Can you work these out from the drawing? Everything is in mm from the part's minimum corner. Round coordinates to 2 decimals unless told otherwise and drop trailing zeros. Loops run counter-clockwise (first coordinate to the right, second up) from the corner with the lowest first, then second, coordinate; pieces in that order, holes last. Notation, with made-up numbers: (-26, -10) -> (-10, -10) arc R21 cw to (-10, 24) -> close; hole circle Ø11 at (38, -14.5). An arc over 180 degrees is marked (long way). Answer as a JSON object with one key per item and string values.
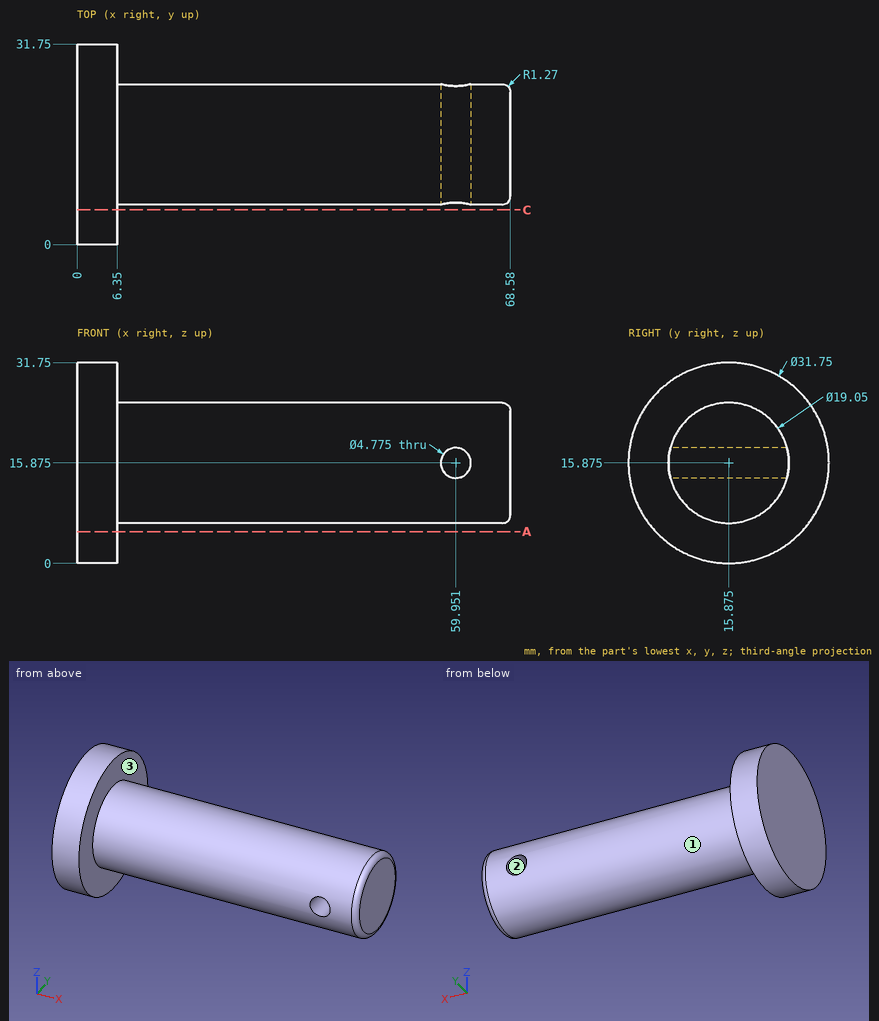
Q1. I'm going to push flat-ended pins straight in: pin 1 (5 mm diameter, centred on x = 18.5, z = 15.5, fed in from +Y); pin 2 (1 mm diameter, centred on x = 23, z = 23, fed in from +Y); pin 3 (4 mm diameter, centred on x = 12, y = 18, fed in from +Z). Where does each tip first touch, or does it pass through?
Determined:
{"pin 1": "y = 25.4", "pin 2": "y = 22.72", "pin 3": "z = 25.4"}
Q2. I want a section at A-A, the plane z = 5. Write out the boundary of the cut face in (x, y).
Determined:
{"outline": "(0, 4.31) -> (6.35, 4.31) -> (6.35, 27.44) -> (0, 27.44) -> close"}
Q3. I want a section at C-C, the plane y = 5.5. Write out the boundary of the cut face in (x, z).
Determined:
{"outline": "(0, 3.86) -> (6.35, 3.86) -> (6.35, 27.89) -> (0, 27.89) -> close"}
Q4. If I drill on L1, parallel to X at y = 23.5, z = 7.5; L2, parallel to Z at x = 36, y = 16; L3, parallel to X at y = 8, z = 13, over which ranges is the centre line in solid material (lowest first)? Write a range as [from, to].
Determined:
{"L1": "[0, 6.35]", "L2": "[6.35, 25.4]", "L3": "[0, 68.57]"}
Q5. We'd pull the mould along Z, two halves only. Please class the marked faces 1, 2 and 3: pulls with the +Z half, pulls with the -Z half, needs draft (parallel to the pull), parting line crosses it, or undercut.
Determined:
{"face 1": "parting line crosses it", "face 2": "undercut", "face 3": "needs draft"}
